Could you check a few things on this model? Use its own coordinates, in mm. A direction names the side the tool comes from. Give positions to 0.01 mm unless a question says otherwise; leave off trailing zeros. Order: outer loops, then holes, each group sorted by start corner. A loop starts at its lowest first (then second) coordinate and runs counter-clockwise, first axis right, second up. Notation, with made-up numbers: M 75,53 L 84,53 A10 cw 84,64 Z; hole C -32.5,56.5 d4. An arc over 180 degrees is marked long. Use a Markdown table: item, result. Add a question column.
```python
from build123d import *

# Parameters (mm, degrees)
PAD004_DEPTH    = 19
SKETCH019_W     = 10
SKETCH019_H     = 3.65
PAD005_DEPTH    = 2
SKETCH020_R     = 1.15
POCKET016_DEPTH = 3.651
CHAMFER001_SIZE = 0.4


with BuildPart() as part:
    # Sketch018 → Pad004 (new body)
    with BuildSketch(Plane.YZ):
        Polygon((-4, 0), (4, 0), (5, -3.65), (-5, -3.65), align=None)
    extrude(amount=PAD004_DEPTH)

    # Sketch019 (on Face5 of Pad004) → Pad005 (join)
    with BuildSketch(Plane(origin=(0, 0, 0), x_dir=(0, 1, 0), z_dir=(-1, 0, 0))):
        with Locations((0, 1.825)):
            Rectangle(SKETCH019_W, SKETCH019_H)
    extrude(amount=-PAD005_DEPTH)

    # Sketch020 (on Face8 of Pad005) → Pocket016 (cut, through all)
    with BuildSketch(Plane(origin=(0, 0, 0), x_dir=(0, -1, 0), z_dir=(0, 0, 1))):
        with Locations((0, 1.75)):
            Circle(SKETCH020_R)
    extrude(amount=-POCKET016_DEPTH, mode=Mode.SUBTRACT)

    # Chamfer001
    chamfer001_edges = [part.edges().sort_by_distance(p)[0] for p in [
        (1.75, 1.15, 0),
    ]]
    chamfer(chamfer001_edges, length=CHAMFER001_SIZE)


with BuildPart() as part_1:
    # Body001 placement: moved
    add(part.part.moved(Location((-10.75, 0, 14))))


solid = part_1.part
```
1) We'd pull the mould along X, two halves only. Please class faces 1 (the face through (-10.75, 0, 12)), 2 (the face through (-10.123, 0.249, 11.998)), 3 (the face through (-8.75, -4.7, 13)), 4 (the face through (-10, -5, 12)): pulls with the +X half, pulls with the -X half, needs draft (parallel to the pull), parting line crosses it, or undercut.
2) Suppose I cut it at B-B on x = -9. Please give me the cut outline in (y, z), and give its area (3 significant figures).
3) Please list where these lines run through material, in increasing order: line 1 (X direction, y = 0, z = 11); line 2 (Y direction, x = -8, z = 13.4); line 3 (X direction, y = -0.5, z = 12.65). Write a range as from..to.
4) Suppose I cut it at C-C on z = 10.8. Please give me the cut outline in (x, y), and give its area (3 significant figures).
5) For pin 1 (1.5 mm diameter, centred on x = 3.5, z = 12.5, fed in from -Y), with a flat end and sliding along its axis, tell me the tip position at first contact or that it passes through.
6) Suppose I cut it at D-D on x = 4. Please give me the cut outline in (y, z), and give its area (4 significant figures).
7) For faces 5 (the face through (-0.369, 4.493, 12.201)), 6 (the face through (-0.369, -4.507, 12.149)), 7 (the face through (-10, 5, 12)), which set-ups out of +Z, -Z, +X, -X, +Y, -Y let a thin tool reach every point of the face, with its end or its side?
8) Suppose I cut it at A-A on y = 0. Please give me the cut outline in (x, z).
Values found:
| question | item | result |
|---|---|---|
| 1 | face 1 | pulls with the -X half |
| 1 | face 2 | undercut |
| 1 | face 3 | pulls with the +X half |
| 1 | face 4 | needs draft |
| 2 | outline | M -5,10.35 L -1.15,10.35 L -1.15,13.6 L -1.55,14 L -5,14 Z; M 1.15,10.35 L 5,10.35 L 5,14 L 1.55,14 L 1.15,13.6 Z |
| 2 | area | 27.9 mm^2 |
| 3 | line 1 | x = -10.75..-10.15, -7.85..8.25 |
| 3 | line 2 | y = -4.16..-0.57, 0.57..4.16 |
| 3 | line 3 | x = -10.75..-10.04, -7.96..8.25 |
| 4 | outline | M -10.75,-5 L -8.75,-5 L -8.75,-4.88 L 8.25,-4.88 L 8.25,4.88 L -8.75,4.88 L -8.75,5 L -10.75,5 Z; hole C -9,0 d2.3 |
| 4 | area | 182 mm^2 |
| 5 | pin 1 | stops at y = -4.62 |
| 6 | outline | M -5,10.35 L 5,10.35 L 4,14 L -4,14 Z |
| 6 | area | 32.85 mm^2 |
| 7 | face 5 | +Z, +X, +Y |
| 7 | face 6 | +Z, +X, -Y |
| 7 | face 7 | +Z, -Z, +X, -X, +Y |
| 8 | outline | M -10.75,10.35 L -10.15,10.35 L -10.15,13.6 L -10.55,14 L -10.75,14 Z; M -7.85,10.35 L 8.25,10.35 L 8.25,14 L -7.45,14 L -7.85,13.6 Z |
